Verification items for the finished model (mm, model axes). Face numbers are marked on the shaded views. Give positions to 0.01 mm unless a question says otherwise; leave off trailing zeros. Write each loop counter-clockwise with the first axis right and the second up, starting at its lowest first coordinate (ties: lowest second). Pieces come first, ordered by that corner, then holes. Notation, with made-up numbers: (-10.75, -24) -> (31.25, -24) arc R20 ccw to (31.25, -18) -> close; hole circle Ø6 at (14.25, -28). An arc over 180 degrees is marked (long way). Answer as CSV lines item,"result".
```python
from build123d import *

# Parameters (mm, degrees)
EXTRUDE_1_DEPTH     = 6
SKETCH_2_R          = 1.6
CUT_EXTRUDE_1_DEPTH = 6
SKETCH_3_R          = 12.5
CUT_EXTRUDE_2_DEPTH = 10


# Read off the part's stored shape, not the designer's step: 凸台-拉伸1
with BuildPart() as part:
    # 凸台-拉伸1 outline → 凸台-拉伸1 (new body)
    with BuildSketch(Plane(origin=(0, 0, 0), x_dir=(1, 0, 0), z_dir=(0, 1, 0))):
        with BuildLine():
            ThreePointArc((-15, 25.980762114), (-21.213203436, -21.213203436), (25.980762114, -15))
            Line((25.980762114, -15), (31.980762114, -15))
            Line((31.980762114, -15), (31.980762114, 15))
            Line((31.980762114, 15), (25.980762114, 15))
            ThreePointArc((25.980762114, 15), (21.213203436, 21.213203436), (15, 25.980762114))
            Line((15, 25.980762114), (15, 35.980762114))
            Line((15, 35.980762114), (-15, 35.980762114))
            Line((-15, 35.980762114), (-15, 25.980762114))
        make_face()
    extrude(amount=EXTRUDE_1_DEPTH)

    # 草图2 → 切除-拉伸1 (cut)
    with BuildSketch(Plane(origin=(0, 6, 0), x_dir=(1, 0, 0), z_dir=(0, 1, 0))):
        with Locations(Location((28.980762114, 10, 0), (0, 0, 270))):
            Circle(SKETCH_2_R)
        with Locations(Location((-15.5, 15.5, 0), (0, 0, 270))):
            Circle(SKETCH_2_R)
        with Locations(Location((15.5, 15.5, 0), (0, 0, 270))):
            Circle(SKETCH_2_R)
        with Locations(Location((-15.5, -15.5, 0), (0, 0, 270))):
            Circle(SKETCH_2_R)
        with Locations(Location((15.5, -15.5, 0), (0, 0, 270))):
            Circle(SKETCH_2_R)
        with Locations(Location((28.980762114, 0, 0), (0, 0, 270))):
            Circle(SKETCH_2_R)
        with Locations(Location((28.980762114, -10, 0), (0, 0, 270))):
            Circle(SKETCH_2_R)
        with Locations(Location((-10, 30.980762114, 0), (0, 0, 270))):
            Circle(SKETCH_2_R)
        with Locations(Location((0, 30.980762114, 0), (0, 0, 270))):
            Circle(SKETCH_2_R)
        with Locations(Location((10, 30.980762114, 0), (0, 0, 270))):
            Circle(SKETCH_2_R)
    extrude(amount=-CUT_EXTRUDE_1_DEPTH, mode=Mode.SUBTRACT)

    # 草图3 → 切除-拉伸2 (cut)
    with BuildSketch(Plane(origin=(0, 6, 0), x_dir=(1, 0, 0), z_dir=(0, 1, 0))):
        with Locations(Location((0, 0, 0), (0, 0, 270))):
            Circle(SKETCH_3_R)
    extrude(amount=-CUT_EXTRUDE_2_DEPTH, mode=Mode.SUBTRACT)


solid = part.part
```
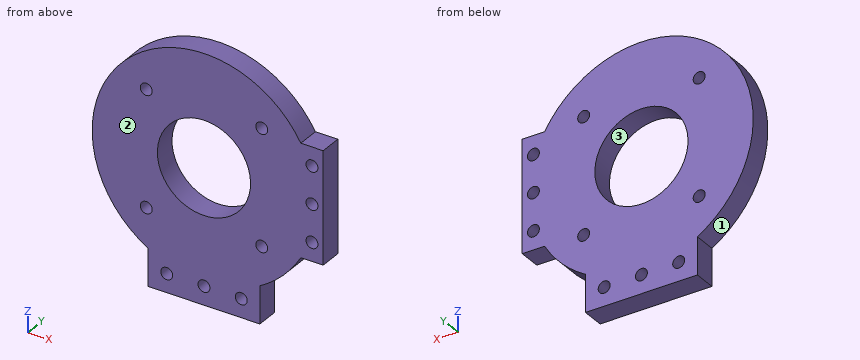
1) Section check B-B (z = 0). Record the boundary of the cut face in (x, y), and give its area (3 significant figures).
Reported:
outline,"(-30, 0) -> (-12.5, 0) -> (-12.5, 6) -> (-30, 6) -> close; (12.5, 0) -> (27.38, 0) -> (27.38, 6) -> (12.5, 6) -> close; (30.58, 0) -> (31.98, 0) -> (31.98, 6) -> (30.58, 6) -> close"
area,"203 mm²"
2) Scan lines: line 1 along X through (y, z) = (4.5, 15.5); line 2 along X through (y, z) = (4.65, 10); line 3 along X through (y, z) = (3.2, -32). Record each from-to range of solid material in increasing order.
Reported:
line 1,"-25.69 to -17.1, -13.9 to 13.9, 17.1 to 25.69"
line 2,"-28.28 to -7.5, 7.5 to 27.38, 30.58 to 31.98"
line 3,"-15 to -11.23, -8.77 to -1.23, 1.23 to 8.77, 11.23 to 15"
3) Draft check along Z on the marked faces 1, 2 and 3. Enter one of: +Z half, -Z half, draft (parallel to the pull), parting line (faces both ways), or undercut.
Reported:
face 1,"parting line"
face 2,"draft"
face 3,"undercut"
4) Section check D-D (z = -24). Record the boundary of the cut face in (x, y).
Reported:
outline,"(-18, 0) -> (18, 0) -> (18, 6) -> (-18, 6) -> close"
5) Section check C-C (y = 2.95). State how many separate pieces and enclosed holes the cut face has, and give its area (3 significant figures).
Reported:
separate pieces,"1"
enclosed holes,"11"
area,"2,570 mm²"
6) Depth check by flat-ended pin: pin 1 (1 mm diameter, centred on x = 11.5, y = 4, fed in from +Z); pin 2 (3 mm diameter, centred on y = 3, z = -28.5, fed in from -X); pin 3 (3 mm diameter, centred on x = 28.5, y = 2, fed in from -Z). Enter the tip coordinate at first touch or a pass-through.
Reported:
pin 1,"z = 27.91"
pin 2,"x = -15"
pin 3,"z = -15"
7) Section check A-A (x = 0). Record the boundary of the cut face in (y, z).
Reported:
outline,"(0, -35.98) -> (6, -35.98) -> (6, -32.58) -> (0, -32.58) -> close; (0, -29.38) -> (6, -29.38) -> (6, -12.5) -> (0, -12.5) -> close; (0, 12.5) -> (6, 12.5) -> (6, 30) -> (0, 30) -> close"
